from build123d import *

# Parameters (mm, degrees)
F0_W     = 50
F0_H     = 50
F1_DEPTH = 25
F2_R     = 16.200601
F3_DEPTH = 40
F4_R     = 13.5
F5_DEPTH = 40


with BuildPart() as f1:
    # F0 (on Front) → F1 (new body)
    with BuildSketch(Plane.XZ):
        with Locations((-0.520919, -0.873815)):
            Rectangle(F0_W, F0_H)
    extrude(amount=F1_DEPTH)

    # F2 (on Front) → F3 (join)
    with BuildSketch(Plane.XZ):
        Circle(F2_R)
    extrude(amount=F3_DEPTH)

    # F4 (on Front) → F5 (cut)
    with BuildSketch(Plane.XZ):
        Circle(F4_R)
    extrude(amount=F5_DEPTH, mode=Mode.SUBTRACT)


solid = f1.part
Could you check a few things on this model? Use its own coordinates, in mm. A direction names the side the tool comes from. Give positions to 0.01 mm unless a question says otherwise; leave off trailing zeros. Order: outer loops, then holes, each group sorted by start corner. A loop starts at its lowest first (then second) coordinate and runs counter-clockwise, first axis right, second up.
1. We'd pull the mould along X, two halves only. Please class faces 3 (the flat face through (-1, -12, 24.126)), 4 (the cylindrical face through (-2.93, -19.72, -13.18)), 5 (the flat face through (24.479, -12, -1)): pulls with the +X half, pulls with the -X half, needs draft (parallel to the pull), parting line crosses it, or undercut.
2. Will these pins go through, and if not, where does the flat tip stop? P1, Ø8, axis at x = -19, y = -28, coming from the +Z side; P2, Ø4, axis at x = 14.5, y = -33.5, coming from the +Z side; P3, Ø5, axis at x = -16.5, z = -10, coming from the -Y side.
3. Suppose I cut it at B-B (x = 0). List the corners of the cut face in (y, z) for me.
4. Suppose I cut it at C-C (y = -8). List the corners of the cut face in (x, z) for me, plus the area to 3 significant figures.
5. Suppose I cut it at D-D (x = -22). List the corners of the cut face in (y, z) for me, plus the area to 3 significant figures.
6. I need wall thicknesses on L1, parallel to Z at x = 0, y = -9.5; L2, parallel to Z at x = 0, y = -26; L3, parallel to Y at x = -19.5, z = -12. Which ranges of each line are inside material? Lowest first, please.
7. For faces 1 (the flat face through (-25.521, -12, -1)), 2 (the cylindrical face through (15.45, -32.39, 4.87)), which set-ups out of +Z, -Z, +X, -X, +Y, -Y let a thin tool reach every point of the face, with its end or its side?
8. Suppose I cut it at A-A (z = 0). List the corners of the cut face in (x, y) for me, plus the area to 3 significant figures.
Solved:
1. face 3: needs draft
1. face 4: undercut
1. face 5: pulls with the +X half
2. P1: stops at z = 24.13
2. P2: stops at z = 10.31
2. P3: stops at y = -25
3. outline: (-40, -16.2) - (-25, -16.2) - (-25, -25.87) - (0, -25.87) - (0, -13.5) - (-40, -13.5) - close; (-40, 13.5) - (0, 13.5) - (0, 24.13) - (-25, 24.13) - (-25, 16.2) - (-40, 16.2) - close
4. outline: (-25.52, -25.87) - (24.48, -25.87) - (24.48, 24.13) - (-25.52, 24.13) - close; hole circle Ø27 at (0, 0)
4. area: 1,930 mm2
5. outline: (-25, -25.87) - (0, -25.87) - (0, 24.13) - (-25, 24.13) - close
5. area: 1,250 mm2
6. L1: z = -25.87 to -13.5, 13.5 to 24.13
6. L2: z = -16.2 to -13.5, 13.5 to 16.2
6. L3: y = -25 to 0
7. face 1: +Z, -Z, -X, +Y, -Y
7. face 2: -Y
8. outline: (-25.52, -25) - (-16.2, -25) - (-16.2, -40) - (-13.5, -40) - (-13.5, 0) - (-25.52, 0) - close; (13.5, -40) - (16.2, -40) - (16.2, -25) - (24.48, -25) - (24.48, 0) - (13.5, 0) - close
8. area: 656 mm2
